Autodesk Inventor part; units mm, degrees
ref_plane "YZ Plane" through (0, 0, 0) normal (1, 0, 0) x (0, 1, 0)
ref_plane "XZ Plane" through (0, 0, 0) normal (0, 1, 0) x (-1, 0, 0)
ref_plane "XY Plane" through (0, 0, 0) normal (0, 0, 1) x (1, 0, 0)
sketch "Base" plane through (0, 0, 0) normal (0, 0, 1) x (1, 0, 0)
  line L0 (-56, 0) -> (56, 0)
  line L1 (0, -56) -> (0, 56) construction
  circle A0 centre (0, 0) radius 40
  line L2 (0, 0) -> (28.2843, 28.2843) construction
  circle A1 centre (28.2843, 28.2843) radius 2.2
  circle A2 centre (-28.2843, 28.2843) radius 2.2
  circle A3 centre (28.2843, -28.2843) radius 2.2
  circle A4 centre (-28.2843, -28.2843) radius 2.2
  circle A5 centre (28.2843, 28.2843) radius 4
  circle A6 centre (-28.2843, 28.2843) radius 4
  circle A7 centre (28.2843, -28.2843) radius 4
  circle A8 centre (-28.2843, -28.2843) radius 4
  circle A9 centre (0, 0) radius 12.2174 construction
  spline S0 degree 3 number of poles 906
  spline S1 degree 3 number of poles 906
  spline S2 degree 3 number of poles 906
  spline S3 degree 3 number of poles 906
  spline S4 degree 2 number of poles 341
  arc A10 (7.6354, -22.3136) -> (7.8387, -21.1617) centre (9.1457, -21.9862) ccw
  circle A11 centre (0, 0) radius 26.5
  point P0 (0, 0)
  point P1 (25.318, 30.9677)
  point P2 (-25.318, 30.9677)
  point P3 (-30.9677, 25.318)
  point P4 (-40, 0)
  point P5 (40, 0)
  point P6 (30.9677, 25.318)
  point P7 (30.9677, -25.318)
  point P8 (-30.9677, -25.318)
  point P9 (-25.318, -30.9677)
  point P10 (25.318, -30.9677)
  point P11 (-29.7965, 26.6864)
  point P12 (-26.6864, 29.7965)
  point P13 (-26.6864, -29.7965)
  point P14 (-29.7965, -26.6864)
extrude "Plate1" add sketch "Base" along normal blind 3 contours A11 L0 A0 A6 A5 | L0 A0 A7 A8 A11 | A5 A0 A1 | A0 A1 A5 | A7 A0 A3 | A0 A3 A7 | A6 A0 A2 | A0 A2 A6 | A8 A0 A4 | A0 A4 A8
fillet "FilletsFeature" radius 6 8 edges at (-30.9677, 25.318, 1.5) (-30.9677, -25.318, 1.5) (-25.318, -30.9677, 1.5) (25.318, -30.9677, 1.5) (30.9677, -25.318, 1.5) (30.9677, 25.318, 1.5) (25.318, 30.9677, 1.5) (-25.318, 30.9677, 1.5)
sketch "WheelEncoderMount" plane through (0, 0, 3) normal (0, 0, 1) x (1, 0, 0)
  circle A0 centre (-20.9919, -21) radius 1.25
  circle A1 centre (-20.9919, 21) radius 1.25
  circle A2 centre (21.0081, -21) radius 1.25
  circle A3 centre (21.0081, 21) radius 1.25
  circle A4 centre (-20.9919, -21) radius 1.25
  circle A5 centre (-20.9919, 21) radius 1.25
hole "EncoderMountHolesFeature" at (-20.9919, -21, 3) at (-20.9919, 21, 3) at (21.0081, 21, 3) at (21.0081, -21, 3) direction (0, 0, -1) diameter 2.45 end through all
equation "\"d48\" = Thickness"
equation "\"d28\" = Thickness"
equation "\"BendRadius\" = Thickness"
equation "\"BendReliefWidth\" = Thickness"
equation "\"BendReliefDepth\" = 0.5 * Thickness"
equation "\"CornerReliefSize\" = 4 * Thickness"
equation "\"MinimumRemnant\" = 2 * Thickness"
equation "\"TransitionRadius\" = BendRadius"
equation "\"JacobiRadiusSize\" = BendRadius"
equation "\"GapSize\" = Thickness"
properties part number "CimCoderMount"
For this review, take the finished solid that the model builds, in its own axes (mm). Coordinates: 2 decimals unless noted, no trailing zeros. Order: outer loops, then holes, each group sorted by start corner. A loop starts at its lowest first (then second) coordinate and runs counter-clockwise, first axis right, second up. Notation, with made-up numbers: (30, -30) - (38, -30) arc R21 ccw to (38, -15) - close; hole circle Ø4 at (10, -29). An arc over 180 degrees is marked (long way). Answer as CSV lines item,"result". Start each with the question number.
1) Insertion check: P1, Ø1.5, axis at y = 19.5, z = 2, coming from the +X side. The pin has a flat end and moves straight along its axis. Give the tip position at first contact, or say it passes through.
2) Add section A-A (x = 0). State the section outline as (y, z) points.
3) Add section C-C (y = -21). State the section outline as (x, z) points, then the cut area to 3 significant figures.
4) Draft analysis for pull direction Y (two halves, no side actions). For faces 1 (the cylindrical face through (0, -40, 1)), 2 (the cylindrical face through (30.38, 27.62, 1.48)), 3 (the flat face through (26, -8, 3)), 4 (the cylindrical face through (-40, 0, 1)), state which applies: +Y half, -Y half, draft (parallel to the pull), parting line (faces both ways), or undercut.
5) To check wall thickness, follow line 1 along Y through (x, z) = (0, 2.2); line 2 along Y through (x, z) = (-20, 0.3); line 3 along Y through (x, z) = (22, 1.6). State the ranges of each line that lie inside material, in increasing order. Write a range as [from, to].
6) Add section D-D (z = 1). Count the separate pieces of the cut face and the enclosed holes in it, then the cut area to 3 significant figures.
Result:
1,P1,"x = 35.33"
2,outline,"(-40, 0) - (-26.5, 0) - (-26.5, 3) - (-40, 3) - close; (26.5, 0) - (40, 0) - (40, 3) - (26.5, 3) - close"
3,outline,"(-34.04, 0) - (-22.22, 0) - (-22.22, 3) - (-34.04, 3) - close; (-19.77, 0) - (-16.16, 0) - (-16.16, 3) - (-19.77, 3) - close; (16.16, 0) - (19.78, 0) - (19.78, 3) - (16.16, 3) - close; (22.23, 0) - (34.04, 0) - (34.04, 3) - (22.23, 3) - close"
3,area,"92.6 mm^2"
4,face 1,"-Y half"
4,face 2,"undercut"
4,face 3,"draft"
4,face 4,"parting line"
5,line 1,"[-40, -26.5], [26.5, 40]"
5,line 2,"[-34.64, -21.72], [-20.28, -17.39], [17.39, 20.28], [21.72, 34.64]"
5,line 3,"[-33.41, -21.72], [-20.28, -14.77], [14.77, 20.28], [21.72, 33.41]"
6,separate pieces,"1"
6,enclosed holes,"9"
6,area,"2,860 mm^2"
